```python
from build123d import *

# Parameters (mm, degrees)
F0_W     = 149.0205824375
F0_H     = 124.2497935891
F1_DEPTH = 91.44
F2_W     = 133.9053437114
F2_H     = 107.7639774892
F3_DEPTH = 91.441
F4_W     = 76.6777545214
F4_H     = 21.7983949804
F5_DEPTH = 25.4
F6_W     = 76.5557736158
F6_H     = 14.9245489264
F7_DEPTH = 25.4
F8_R     = 10.6028855258
F9_DEPTH = 149.0215824375


with BuildPart() as f1:
    # F0 (on Top) → F1 (new body)
    with BuildSketch(Plane.XY):
        Rectangle(F0_W, F0_H)
    extrude(amount=F1_DEPTH)

    # F2 (on face) → F3 (cut, through all)
    with BuildSketch(Plane.XY.offset(91.44)):
        with Locations((-0.2857260406, 1.6505084932)):
            Rectangle(F2_W, F2_H)
    extrude(amount=-F3_DEPTH, mode=Mode.SUBTRACT)

    # F4 (on face) → F5 (cut)
    with BuildSketch(Plane.XZ.offset(62.1248967946)):
        with Locations((-0.7736906409, 80.5408025098)):
            Rectangle(F4_W, F4_H)
    extrude(amount=-F5_DEPTH, mode=Mode.SUBTRACT)

    # F6 (on face) → F7 (cut)
    with BuildSketch(Plane(origin=(0, 62.1248967946, 0), x_dir=(-1, 0, 0), z_dir=(0, 1, 0))):
        with Locations((3.8653835654, 83.9777255368)):
            Rectangle(F6_W, F6_H)
    extrude(amount=-F7_DEPTH, mode=Mode.SUBTRACT)

    # F8 (on face) → F9 (cut, through all)
    with BuildSketch(Plane.YZ.offset(74.5102912188)):
        with Locations((0, 48.8554276526)):
            Circle(F8_R)
    extrude(amount=-F9_DEPTH, mode=Mode.SUBTRACT)


solid = f1.part
```
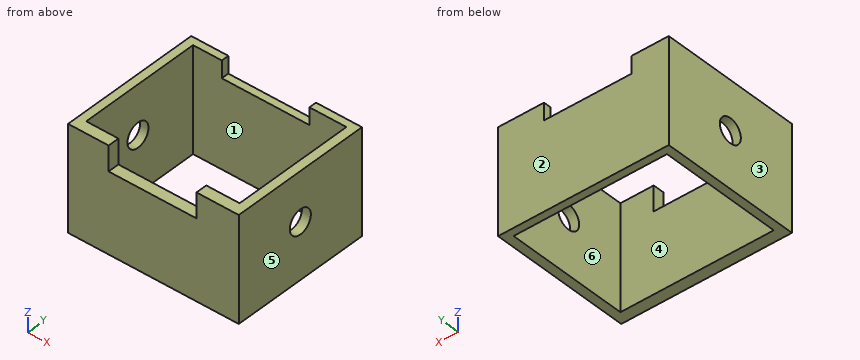
Model file for the job. Use its own axes, mm. Face numbers are marked on the shaded views. A direction names the side the tool comes from. Round coordinates to 2 decimals unless told otherwise and drop trailing zeros. Write each loop counter-clockwise with the first axis right and the second up, starting at its lowest first coordinate (ties: lowest second). Pieces come first, ordered by that corner, then holes. Notation, with made-up numbers: M 86.5,59 L 90.5,59 A15 cw 90.5,76 Z; hole C 72,43.5 d9. An arc over 180 degrees is marked long. Put each result on its own line as item: value.
Item 1: Cut at A-A (y = 22.5). List the corners of the cut face in (x, z), and give its area (3 significant figures).
Responses:
outline: M -74.51,0 L -67.24,0 L -67.24,91.44 L -74.51,91.44 Z; M 66.67,0 L 74.51,0 L 74.51,91.44 L 66.67,91.44 Z
area: 1,380 mm²
Item 2: Tool access for the marked faces 5 and 6: list every direction of +Z, -Z, +X, -X, +Y, -Y with a clear straight run to the whole face (end or side of a thin tool).
Responses:
face 5: +Z, -Z, +X, +Y, -Y
face 6: +Z, -Z
Item 3: Flat gauge pins, fed straight in: P1, Ø3, axis at x = -14, y = -58.5, coming from the +Z side; P2, Ø7.5, axis at x = -15, y = 60, coming from the +Z side. Where does each tip first touch, or does it go through?
Responses:
P1: z = 69.64
P2: z = 76.52
Item 4: Cut at C-C (z = 22). List the corners of the cut face in (x, y), and give its area (3 significant figures).
Responses:
outline: M -74.51,-62.12 L 74.51,-62.12 L 74.51,62.12 L -74.51,62.12 Z; hole M -67.24,-52.23 L 66.67,-52.23 L 66.67,55.53 L -67.24,55.53 Z
area: 4,090 mm²
Item 5: Cut at B-B (x = -44). List the corners of the cut face in (y, z), and give its area (3 significant figures).
Responses:
outline: M -62.12,0 L -52.23,0 L -52.23,91.44 L -62.12,91.44 Z; M 55.53,0 L 62.12,0 L 62.12,91.44 L 55.53,91.44 Z
area: 1,510 mm²
Item 6: Probe L1, parallel to X at y = 2, z = 30.5; L2, parallel to Y at x = -61, z = 12; L3, parallel to Z at x = -70, y = 0. List the from-to ranges inside material, lowest first. Write a range as from..to.
Responses:
L1: -74.51..-67.24, 66.67..74.51
L2: -62.12..-52.23, 55.53..62.12
L3: 0..38.25, 59.46..91.44
Item 7: Cut at D-D (y = 0). List the corners of the cut face in (x, z).
Responses:
outline: M -74.51,0 L -67.24,0 L -67.24,38.25 L -74.51,38.25 Z; M -74.51,59.46 L -67.24,59.46 L -67.24,91.44 L -74.51,91.44 Z; M 66.67,0 L 74.51,0 L 74.51,38.25 L 66.67,38.25 Z; M 66.67,59.46 L 74.51,59.46 L 74.51,91.44 L 66.67,91.44 Z
Item 8: Mould opens along Y. For the marked faces 1, 2, 3 and 4 say: +Y half, -Y half, draft (parallel to the pull), parting line (faces both ways), or undercut.
Responses:
face 1: undercut
face 2: +Y half
face 3: draft
face 4: undercut
